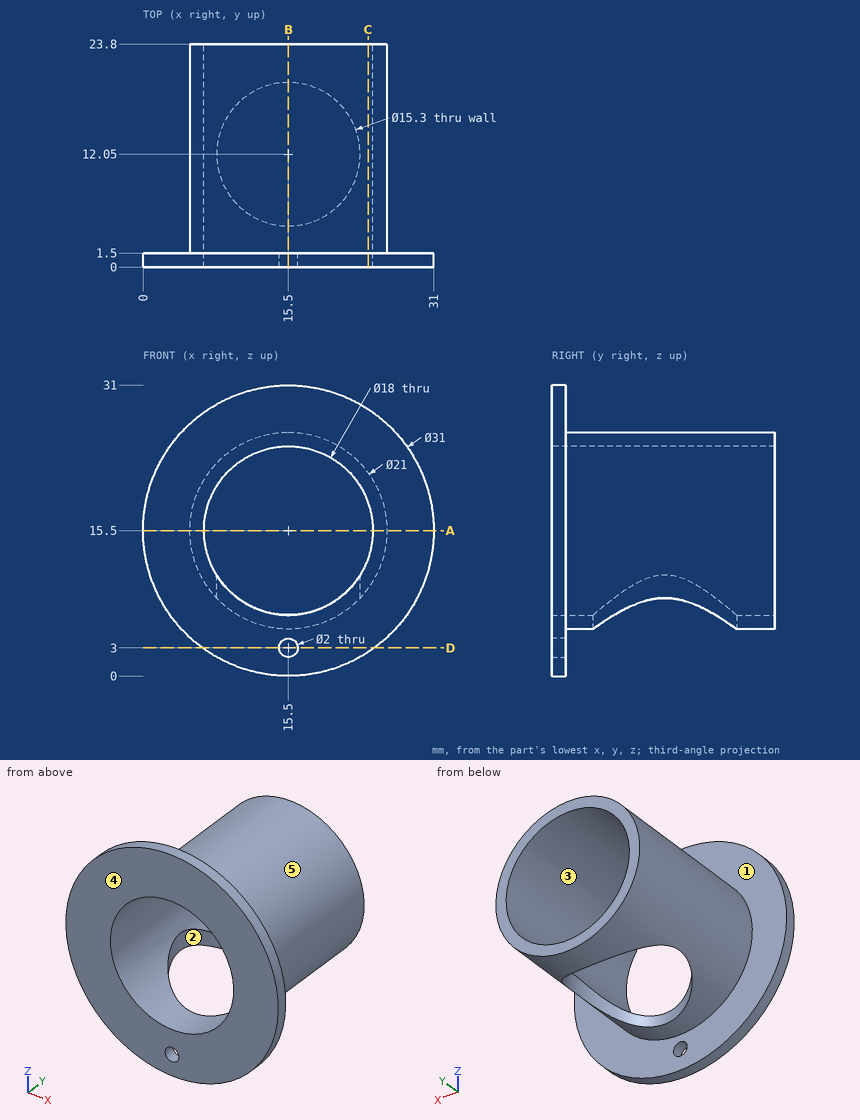
The figure shows three views and two pictorial views of one solid part (mm, origin at its lowest corner). Answer the questions. A direction names the side the tool comes from. Give positions to 0.01 mm unless a question says otherwise; leave off trailing zeros. Write each loop counter-clockwise with the first axis right and the second up, starting at its lowest first coordinate (ties: lowest second). Pieces come first, ordered by that corner, then holes.
Q1. The part is cut by section A-A on z = 15.5. Give the vertices of the cut face in (x, y), and give its area (3 significant figures).
Answer:
outline: (0, 0) - (6.5, 0) - (6.5, 23.8) - (5, 23.8) - (5, 1.5) - (0, 1.5) - close; (24.5, 0) - (31, 0) - (31, 1.5) - (26, 1.5) - (26, 23.8) - (24.5, 23.8) - close
area: 86.4 mm2
Q2. Straight lines are drawn through the part: L1, parallel to X at y = 6.5, z = 15.5; L2, parallel to Y at x = 8.5, z = 2.5; L3, parallel to Z at x = 15.5, y = 13. For each, find the intervals that lie inside material, in ascending order.
Answer:
L1: x = 5 to 6.5, 24.5 to 26
L2: y = 0 to 1.5
L3: z = 24.5 to 26
Q3. For a pull along Z with two mould halves and no side action, classify the marked faces 3, 4 and 5 as released by +Z, released by -Z, zero draft, split by the parting line, or undercut.
Answer:
face 3: undercut
face 4: zero draft
face 5: split by the parting line
Q4. The part is cut by section B-B on x = 15.5. Give the vertices of the cut face in (y, z), and give its area (4 significant figures).
Answer:
outline: (0, 0) - (1.5, 0) - (1.5, 2) - (0, 2) - close; (0, 4) - (1.5, 4) - (1.5, 5) - (4.4, 5) - (4.4, 6.5) - (0, 6.5) - close; (0, 24.5) - (23.8, 24.5) - (23.8, 26) - (1.5, 26) - (1.5, 31) - (0, 31) - close; (19.7, 5) - (23.8, 5) - (23.8, 6.5) - (19.7, 6.5) - close
area: 60.45 mm2
Q5. The part is cut by section C-C on x = 24. Give the vertices of the cut face in (y, z), and give its area (3 significant figures).
Answer:
outline: (0, 2.54) - (1.5, 2.54) - (1.5, 9.34) - (23.8, 9.34) - (23.8, 12.54) - (0, 12.54) - close; (0, 18.46) - (23.8, 18.46) - (23.8, 21.66) - (1.5, 21.66) - (1.5, 28.46) - (0, 28.46) - close
area: 173 mm2
Q6. A tool of negligible diameter and unlimited length cuts with its end or side. For the marked faces 1 and 2, from which of +Z, -Z, +X, -X, +Y, -Y can it reach the whole face along a straight path? Write none if from no direction.
Answer:
face 1: +Y
face 2: -Z
Q7. Given pin 1 (1 mm diameter, centred on x = 7.5, y = 21.5, fed in from -Z); pin 2 (5 mm diameter, centred on x = 6, y = 14, fed in from +Z); pin 3 (12 mm diameter, centred on x = 24, y = 13, fed in from +Z), each flat-ended and moving along its own axis, determine where each tip first touches the part or whether it passes through.
Answer:
pin 1: stops at z = 8.15
pin 2: stops at z = 23.33
pin 3: stops at z = 25.7
Q8. The part is cut by section D-D on z = 3. Give the vertices of the cut face in (x, y).
Answer:
outline: (6.33, 0) - (14.5, 0) - (14.5, 1.5) - (6.33, 1.5) - close; (16.5, 0) - (24.67, 0) - (24.67, 1.5) - (16.5, 1.5) - close
